Build history of the part. All positions in model axes, mm. A direction names the side the tool comes from. Round coordinates to 2 decimals unless told otherwise and drop trailing zeros. Write each loop counter-clockwise with the first axis right and the second up, starting at its lowest first coordinate (ties: lowest second). Pieces come first, ordered by that corner, then holes. Notation, with made-up numbers: (-26.75, 77) -> (-5.75, 77) arc R34 ccw to (-5.75, 112) -> close; hole circle Ø4 at (-12, -9.5). An arc over 180 degrees is marked (long way). Answer in a Markdown table with one row per item.
```python
from build123d import *

# Parameters (mm, degrees)
SKETCH1_W           = 20
SKETCH1_H           = 20
SKETCH1_R           = 5.3
BOSS_EXTRUDE1_DEPTH = 35
SKETCH2_W           = 20
SKETCH2_H           = 20
BOSS_EXTRUDE2_DEPTH = 25
CUT_EXTRUDE2_REACH  = 68.332
SKETCH5_R           = 1.5
FILLET2_R           = 10
SKETCH4_W           = 20
SKETCH4_H           = 7.5
CUT_EXTRUDE3_DEPTH  = 21
FILLET3_R           = 5
SKETCH6_W           = 5.65
SKETCH6_H           = 2.5
CUT_EXTRUDE4_DEPTH  = 8
CHAMFER1_SIZE       = 1


with BuildPart() as part:
    # Sketch1 → Boss-Extrude1 (new body)
    with BuildSketch(Plane.XY):
        with Locations((10, 10)):
            Rectangle(SKETCH1_W, SKETCH1_H)
        with Locations((10, 10)):
            Circle(SKETCH1_R, mode=Mode.SUBTRACT)
    extrude(amount=BOSS_EXTRUDE1_DEPTH)

    # Sketch2 → Boss-Extrude2 (add)
    with BuildSketch(Plane.XY.offset(35)):
        with Locations((10, 10)):
            Rectangle(SKETCH2_W, SKETCH2_H)
    extrude(amount=BOSS_EXTRUDE2_DEPTH)

    # Cut-Extrude2: up to this face of the body (flat: up to its plane)
    cut_extrude2_end = Plane(part.part.faces().sort_by_distance((10, 0, 30))[0])
    # Sketch5 → Cut-Extrude2 (cut, up to the picked face)
    with BuildSketch(Plane(origin=(0, 20, 0), x_dir=(1, 0, 0), z_dir=(0, 1, 0)), mode=Mode.PRIVATE) as cut_extrude2_sk1:
        with Locations(Location((10, -5, 0), (0, 0, 270))):
            Circle(SKETCH5_R)
    cut_extrude2_tool1 = split(extrude(cut_extrude2_sk1.sketch, amount=-CUT_EXTRUDE2_REACH, mode=Mode.PRIVATE), bisect_by=cut_extrude2_end, keep=Keep.BOTH, mode=Mode.PRIVATE)
    # Sketch5 → Cut-Extrude2 (cut, up to the picked face)
    with BuildSketch(Plane(origin=(0, 20, 0), x_dir=(1, 0, 0), z_dir=(0, 1, 0)), mode=Mode.PRIVATE) as cut_extrude2_sk2:
        with Locations(Location((10, -50, 0), (0, 0, 270))):
            Circle(SKETCH5_R)
    cut_extrude2_tool2 = split(extrude(cut_extrude2_sk2.sketch, amount=-CUT_EXTRUDE2_REACH, mode=Mode.PRIVATE), bisect_by=cut_extrude2_end, keep=Keep.BOTH, mode=Mode.PRIVATE)
    add(cut_extrude2_tool1.solids().sort_by(Axis((10, 20, 5), (0, -1, 0)))[0], mode=Mode.SUBTRACT)
    add(cut_extrude2_tool2.solids().sort_by(Axis((10, 20, 50), (0, -1, 0)))[0], mode=Mode.SUBTRACT)

    # Fillet2
    fillet2_edges = [part.edges().sort_by_distance(p)[0] for p in [
        (0, 10, 60),
        (20, 10, 60),
    ]]
    fillet(fillet2_edges, radius=FILLET2_R - 0.0001)  # a hair under: the kernel refuses the full size

    # Sketch4 → Cut-Extrude3 (cut)
    with BuildSketch(Plane.XY.offset(60)):
        with Locations((10, 3.75)):
            Rectangle(SKETCH4_W, SKETCH4_H)
        with Locations((10, 16.25)):
            Rectangle(SKETCH4_W, SKETCH4_H)
    extrude(amount=-CUT_EXTRUDE3_DEPTH, mode=Mode.SUBTRACT)

    # Fillet3
    fillet3_edges = [part.edges().sort_by_distance(p)[0] for p in [
        (0, 20, 19.5),
        (20, 20, 19.5),
        (20, 0, 19.5),
        (0, 0, 19.5),
    ]]
    fillet(fillet3_edges, radius=FILLET3_R)

    # Sketch6 → Cut-Extrude4 (cut)
    with BuildSketch(Plane(origin=(0, 0, 0), x_dir=(-1, 0, 0), z_dir=(0, 0, -1))):
        with Locations((-10, 17.5)):
            Rectangle(SKETCH6_W, SKETCH6_H)
        with Locations((-10, 2.5)):
            Rectangle(SKETCH6_W, SKETCH6_H)
    extrude(amount=-CUT_EXTRUDE4_DEPTH, mode=Mode.SUBTRACT)

    # Chamfer1
    chamfer1_edges = [part.edges().sort_by_distance(p)[0] for p in [
        (12.825, 17.5, 8),
        (7.175, 17.5, 8),
        (12.825, 2.5, 8),
        (7.175, 2.5, 8),
    ]]
    chamfer(chamfer1_edges, length=CHAMFER1_SIZE)


solid = part.part
```
Q1. Which spindle directions (+Z, -Z, +X, -X, +Y, -Y) get a long thin tool onto all of the face, cutting with end or side? Do faces 1 (the flat face through (10, 16, 39)), 2 (the flat face through (5, 15, 0)), 3 (the flat face through (10, 16.25, 3)). Say none if no direction does.
A:
| item | result |
|---|---|
| face 1 | +Z, +X, -X, +Y |
| face 2 | -Z, +X, -X, +Y, -Y |
| face 3 | -Z |
Q2. Wall check: line 1 (X direction, y = 10.3, z = 50); line 2 (Z direction, x = 10, y = 4.5); line 3 (Z direction, x = 18, y = 16.25). Give the ranges that are in metal, low to high. Write a range as [from, to].
A:
| item | result |
|---|---|
| line 1 | [0, 8.5], [11.5, 20] |
| line 2 | [0, 3.5], [6.5, 39] |
| line 3 | [0, 39] |
Q3. Saw through at C-C on z = 14.5. Write the cut outline in (x, y).
A:
| item | result |
|---|---|
| outline | (0, 5) arc R5 ccw to (5, 0) -> (15, 0) arc R5 ccw to (20, 5) -> (20, 15) arc R5 ccw to (15, 20) -> (5, 20) arc R5 ccw to (0, 15) -> close; hole circle Ø10.6 at (10, 10) |
Q4. Drop flat-ended pins along their axis: P1, Ø2, axis at x = 13, y = 17.5, coming from the +Z side; P2, Ø2, axis at y = 2, z = 3.5, coming from the -X side; P3, Ø1, axis at x = 9, z = 46, coming from the +Y side. Give the stop position or say it passes through.
A:
| item | result |
|---|---|
| P1 | z = 39 |
| P2 | x = 0.42 |
| P3 | y = 12.5 |
Q5. Two-plate mould, pull along X, no slides. Class faces 4 (the cylindrical face through (16.99, 10.04, 57.15)), 5 (the flat face through (10, 0, 19)), 6 (the flat face through (7.682, 2.482, 7.507)): released by +X, released by -X, zero draft, split by the parting line, or undercut.
A:
| item | result |
|---|---|
| face 4 | released by +X |
| face 5 | zero draft |
| face 6 | undercut |
Q6. Saw through at D-D on x = 16.5. Write the cut outline in (y, z).
A:
| item | result |
|---|---|
| outline | (0.23, 0) -> (19.77, 0) -> (19.77, 39) -> (12.5, 39) -> (12.5, 57.6) -> (7.5, 57.6) -> (7.5, 39) -> (0.23, 39) -> close |
